Autodesk Inventor part; units mm, degrees
ref_plane "YZ Plane" through (0, 0, 0) normal (1, 0, 0) x (0, 1, 0)
ref_plane "XZ Plane" through (0, 0, 0) normal (0, 1, 0) x (-1, 0, 0)
ref_plane "XY Plane" through (0, 0, 0) normal (0, 0, 1) x (1, 0, 0)
sketch "Sketch1" plane through (0, 0, 0) normal (0, 1, 0) x (-1, 0, 0)
  line L0 (16.25, 48.5) -> (-16.25, 48.5)
  line L1 (-16.25, 48.5) -> (-16.25, -48.5)
  line L2 (-16.25, -48.5) -> (16.25, -48.5)
  line L3 (16.25, -48.5) -> (16.25, 48.5)
  line L4 (16.25, 48.5) -> (-16.25, -48.5) construction
  line L5 (-16.25, 48.5) -> (16.25, -48.5) construction
  line L6 (16.25, 48.5) -> (16.25, 40.5)
  line L7 (16.25, -48.5) -> (16.25, -40.5)
  line L8 (16.25, 40.5) -> (-16.25, 40.5)
  line L9 (16.25, -40.5) -> (-16.25, -40.5)
  line L10 (0, 48.5) -> (0, 42.5)
  line L11 (-16.25, 48.5) -> (-10.25, 48.5)
  line L12 (-10.25, 48.5) -> (-10.25, 42.5)
  line L13 (-10.25, 42.5) -> (-16.25, 42.5)
  line L14 (-16.25, 42.5) -> (-16.25, 48.5)
  line L15 (16.25, 48.5) -> (10.25, 48.5)
  line L16 (10.25, 48.5) -> (10.25, 42.5)
  line L17 (10.25, 42.5) -> (16.25, 42.5)
  line L18 (16.25, 42.5) -> (16.25, 48.5)
  line L19 (10.25, 42.5) -> (-10.25, 42.5)
  point P0 (0, 0)
  dimension "d0" = 32.5
  dimension "d1" = 97
  dimension "d4" = 6
  dimension "d5" = 6
  dimension "d6" = 6
  dimension "d7" = 6
  dimension "d8" = 6
extrude "Extrusion1" add sketch "Sketch1" along normal blind 10 contours L3 L17 L16 L0 | L3 L8 L1 L13 L19 L17 | L12 L13 L1 L0 | L3 L2 L1 L9
sketch "Sketch2" plane through (-16.25, 0, -40.5) normal (0, 0, 1) x (1, 0, 0)
  line L0 (0, 10) -> (32.5, 10)
  line L1 (32.5, 10) -> (26.5, 10)
  line L2 (26.5, 10) -> (26.5, 4)
  line L3 (26.5, 4) -> (32.5, 4)
  line L4 (32.5, 4) -> (32.5, 10)
  line L5 (0, 0) -> (0, 10)
  line L6 (0, 10) -> (6, 10)
  line L7 (6, 10) -> (6, 4)
  line L8 (6, 4) -> (0, 4)
  line L9 (0, 4) -> (0, 10)
  point P0 (16.25, 0)
  dimension "d11" = 6
  dimension "d12" = 6
  dimension "d15" = 6
  dimension "d16" = 6
extrude "Extrusion2" add sketch "Sketch2" along normal up to surface (81 mm away)
sketch "Sketch3" plane through (-16.25, 0, -48.5) normal (-1, 0, 0) x (0, 0, 1)
  circle A0 centre (85, 7) radius 1.85
  circle A1 centre (12, 7) radius 1.85
  line L0 (8, 4) -> (89, 4)
  line L1 (97, 0) -> (97, 10)
  line L2 (0, 0) -> (0, 10)
  point P0 (48.5, 0)
  dimension "d17" = 3.7
  dimension "d18" = 3.7
  dimension "d19" = 3
  dimension "d20" = 3
  dimension "d21" = 12
  dimension "d22" = 12
extrude "Extrusion3" cut sketch "Sketch3" against normal up to surface (32.5 mm away)
sketch "Sketch4" plane through (0, 0, 0) normal (0, -1, 0) x (1, 0, 0)
  circle A0 centre (13.75, 46) radius 1.85
  circle A1 centre (13.75, -46) radius 1.85
  circle A2 centre (-13.75, -46) radius 1.85
  circle A3 centre (-13.75, 46) radius 1.85
  line L0 (10.25, 48.5) -> (16.25, 48.5)
  line L1 (16.25, 48.5) -> (16.25, 40.5)
  line L2 (-16.25, 48.5) -> (-10.25, 48.5)
  line L3 (-16.25, 40.5) -> (-16.25, 48.5)
  line L4 (16.25, -40.5) -> (16.25, -48.5)
  line L5 (16.25, -48.5) -> (-16.25, -48.5)
  line L6 (-16.25, -48.5) -> (-16.25, -40.5)
  point P0 (0, 0)
  point P1 (16.25, 44.5)
  dimension "d25" = 3.7
  dimension "d26" = 3.7
  dimension "d27" = 3.7
  dimension "d28" = 3.7
  dimension "d29" = 2.5
  dimension "d30" = 2.5
  dimension "d31" = 2.5
  dimension "d32" = 2.5
  dimension "d33" = 2.5
  dimension "d34" = 2.5
  dimension "d35" = 2.5
  dimension "d36" = 2.5
extrude "Extrusion4" cut sketch "Sketch4" against normal blind 10
equation "\"d18\" = d17"
equation "\"d20\" = d19"
equation "\"d31\" = d29"
equation "\"d32\" = d29"
equation "\"d33\" = d29"
equation "\"d34\" = d29"
equation "\"d35\" = d29"
equation "\"d36\" = d29"
properties part number "V1 screen holder_3DPrint"
Part model, mm, in its own coordinate system. A direction names the side the tool comes from. Coordinates: 2 decimals unless noted, no trailing zeros. Write each loop counter-clockwise with the first axis right and the second up, starting at its lowest first coordinate (ties: lowest second). Pieces come first, ordered by that corner, then holes. Notation, with made-up numbers: M 23,10 L 59,10 A14 cw 59,17 Z; hole C -40,45 d1. An arc over 180 degrees is marked long. Return JSON: item names as keys, results as strings.
1. Saw through at B-B, the plane z = 36.5. Write the cut outline in (x, y), then the cut area to 3 significant figures.
Determined:
{"outline": "M -16.25,4 L -10.25,4 L -10.25,5.15 L -16.25,5.15 Z; M -16.25,8.85 L -10.25,8.85 L -10.25,10 L -16.25,10 Z; M 10.25,4 L 16.25,4 L 16.25,5.15 L 10.25,5.15 Z; M 10.25,8.85 L 16.25,8.85 L 16.25,10 L 10.25,10 Z", "area": "27.6 mm²"}
2. 3-axis set-ups, long thin cutter, end or side, ignore diameter. For faces 5 (the face through (13, 4, -1)), 6 (the face through (10.25, 7, -1)), 7 (the face through (10.25, 5, 46)), 8 (the face through (0, 4, -40.5)): which of +Z, -Z, +X, -X, +Y, -Y reach the whole face in a straight line?
Determined:
{"face 5": "+X, -X, -Y", "face 6": "+Y, -Y", "face 7": "+Z, +Y, -Y", "face 8": "-Y"}
3. Pull direction Y, two halves, no side cores. Call faces 1 (the face through (-13.292, 8.25, -37.864)), 2 (the face through (-13, 4, -1)), 3 (the face through (11, 10, 1)), 4 (the face through (14.604, 4.93, -47.641)): pulls with the +Y half, pulls with the -Y half, needs draft (parallel to the pull), parting line crosses it, or undercut.
Determined:
{"face 1": "undercut", "face 2": "pulls with the -Y half", "face 3": "pulls with the +Y half", "face 4": "needs draft"}
4. Saw through at C-C, the plane x = 13.75. Write the cut outline in (y, z).
Determined:
{"outline": "M 0,-48.5 L 10,-48.5 L 10,-47.85 L 0,-47.85 Z; M 0,-44.15 L 10,-44.15 L 10,44.15 L 0,44.15 L 0,40.5 L 4,40.5 L 4,-40.5 L 0,-40.5 Z; M 0,47.85 L 10,47.85 L 10,48.5 L 0,48.5 Z; hole C 7,-36.5 d3.7; hole C 7,36.5 d3.7"}
5. Flat gauge pins, fed straight in: pin 1 Ø6 at (x, y) = (-1, 9) entering from +Z; pin 2 Ø2 at (x, z) = (-13.75, 46) entering from -Y; pin 3 Ø3 at (x, z) = (-12, 5.5) entering from -Y. Where does each tip first touch, or does it go through?
Determined:
{"pin 1": "z = 42.5", "pin 2": "through", "pin 3": "y = 4"}
6. Saw through at A-A, the plane y = 7. Count the separate pieces of the cut face and the enclosed holes in it, then the cut area to 3 significant figures.
Determined:
{"separate pieces": "4", "enclosed holes": "4", "area": "1,240 mm²"}
7. Probe L1, parallel to Z at x = -14, y = 6.75; L2, parallel to Z at x = -1.5, y = 2.5; L3, parallel to X at y = 5, z = 17.5. List the from-to ranges inside material, lowest first.
Determined:
{"L1": "-48.5 to -47.83, -44.17 to -38.33, -34.67 to 34.67, 38.33 to 44.17, 47.83 to 48.5", "L2": "-48.5 to -40.5, 40.5 to 42.5", "L3": "-16.25 to -10.25, 10.25 to 16.25"}
8. Saw through at D-D, the plane y = 2. Write the cut outline in (x, z), then the cut area to 3 significant figures.
Determined:
{"outline": "M -16.25,-48.5 L 16.25,-48.5 L 16.25,-40.5 L -16.25,-40.5 Z; M -16.25,40.5 L 16.25,40.5 L 16.25,48.5 L 10.25,48.5 L 10.25,42.5 L -10.25,42.5 L -10.25,48.5 L -16.25,48.5 Z; hole C -13.75,-46 d3.7; hole C -13.75,46 d3.7; hole C 13.75,-46 d3.7; hole C 13.75,46 d3.7", "area": "354 mm²"}
